from build123d import *

# Parameters (mm, degrees)
F1_DEPTH = 63.5
F2_W     = 38.1
F2_H     = 12.7
F3_DEPTH = 27.583812
F4_W     = 38.1
F4_H     = 12.7
F5_DEPTH = 25.401


with BuildPart() as f1:
    # F0 (on Front) → F1 (new body)
    with BuildSketch(Plane.XZ):
        Polygon((-30.102565, 39.520449), (-57.685377, 39.520449), (-57.685377, -23.979551), (31.214621, -23.979551), (31.214621, 1.420449), (-30.102565, 1.420449), align=None)
    extrude(amount=F1_DEPTH)

    # F2 (on face) → F3 (cut, through all)
    with BuildSketch(Plane.YZ.offset(-30.102565)):
        with Locations((-31.75, 33.170449)):
            Rectangle(F2_W, F2_H)
    extrude(amount=-F3_DEPTH, mode=Mode.SUBTRACT)

    # F4 (on face) → F5 (cut, through all)
    with BuildSketch(Plane.XY.offset(1.420449)):
        with Locations((12.164621, -31.75)):
            Rectangle(F4_W, F4_H)
    extrude(amount=-F5_DEPTH, mode=Mode.SUBTRACT)


solid = f1.part
Input: part model. Units: mm. Frame: model coordinates. A direction names the side the tool comes from. Round coordinates to 2 decimals unless told otherwise and drop trailing zeros. Order: outer loops, then holes, each group sorted by start corner. A loop starts at its lowest first (then second) coordinate and runs counter-clockwise, first axis right, second up.
1. Mould query, pull axis Y, two halves, no side actions, for faces 1 (the face through (-44, -50.8, 33)), 2 (the face through (1, -24, 1.42)), 3 (the face through (-24, -63.5, 1)). Classes: released by +Y, released by -Y, zero draft, split by the parting line, or undercut.
The answers:
face 1: undercut
face 2: zero draft
face 3: released by -Y
2. Cut plane C-C, the plane y = -27. Output: boundary loops of the cut face in (x, z).
The answers:
outline: (-57.69, -23.98) - (-6.89, -23.98) - (-6.89, 1.42) - (-30.1, 1.42) - (-30.1, 26.82) - (-57.69, 26.82) - close
3. Cut plane A-A, the plane x = 22.5. Output: boundary loops of the cut face in (y, z).
The answers:
outline: (-63.5, -23.98) - (-38.1, -23.98) - (-38.1, 1.42) - (-63.5, 1.42) - close; (-25.4, -23.98) - (0, -23.98) - (0, 1.42) - (-25.4, 1.42) - close
4. Pin query (flat end, axial travel): P1, Ø12.5, axis at x = 21, z = -15.5, coming from the +Y side; P2, Ø3, axis at y = -51, z = 16, coming from the +X side; P3, Ø6.5, axis at y = -33.5, z = -9.5, coming from the +X side; P4, Ø2, axis at x = -23, y = -25, coming from the +Z side. Return the tip coordinate at first contact, or that it passes through.
The answers:
P1: stops at y = 0
P2: stops at x = -30.1
P3: stops at x = -6.89
P4: stops at z = 1.42
5. Cut plane B-B, the plane z = 28.5. Output: boundary loops of the cut face in (x, y), then the cut area to 3 significant figures.
The answers:
outline: (-57.69, -63.5) - (-30.1, -63.5) - (-30.1, -50.8) - (-57.69, -50.8) - close; (-57.69, -12.7) - (-30.1, -12.7) - (-30.1, 0) - (-57.69, 0) - close
area: 701 mm2
6. Material intervals for line 1 (Y direction, x = 0, z = -12.5); line 2 (Y direction, x = -50.5, z = 28); line 3 (Z direction, x = 23.5, y = -60), sorted ascending.
The answers:
line 1: y = -63.5 to -38.1, -25.4 to 0
line 2: y = -63.5 to -50.8, -12.7 to 0
line 3: z = -23.98 to 1.42
7. Set-up query: faces 4 (the face through (-30.103, -31, 16)), 5 (the face through (12, -25.4, -11)), 6 (the face through (-44, -32, 26.82)). Return all of +Z, -Z, +X, -X, +Y, -Y with unobstructed straight access to the full face (end or side cutting, diameter ignored); none if empty.
The answers:
face 4: +Z, +X, +Y, -Y
face 5: +Z, -Z, +X
face 6: +Z, +X, -X
8. Cut plane D-D, the plane x = -46. Output: boundary loops of the cut face in (y, z).
The answers:
outline: (-63.5, -23.98) - (0, -23.98) - (0, 39.52) - (-12.7, 39.52) - (-12.7, 26.82) - (-50.8, 26.82) - (-50.8, 39.52) - (-63.5, 39.52) - close
